```python
from build123d import *

# Parameters (mm, degrees)
F1_DEPTH = 40.2336
F0_R     = 10.16
F2_DEPTH = 15.7734
F3_R     = 3.302


# Not quite as in the source:
# - a feature names something its author has since deleted; it is built from what else it names


with BuildPart() as f1:
    # F0 (on Top) → F1 (new body)
    with BuildSketch(Plane.XY):
        with BuildLine():
            ThreePointArc((5.2118165727, -28.0956863773), (21.9710978739, -18.2702348977), (28.575, 0))
            ThreePointArc((28.575, 0), (21.9710978739, 18.2702348977), (5.2118165727, 28.0956863773))
            ThreePointArc((5.2118165727, 28.0956863773), (-28.575, 0), (5.2118165727, -28.0956863773))
        make_face()
        with BuildLine():
            ThreePointArc((13.4477648793, -4.826), (-14.2875, 0), (13.4477648793, 4.826))
            Line((13.4477648793, 4.826), (19.7977648793, 4.826))
            Line((19.7977648793, 4.826), (19.7977648793, -4.826))
            Line((19.7977648793, -4.826), (13.4477648793, -4.826))
        make_face(mode=Mode.SUBTRACT)
    extrude(amount=F1_DEPTH)

    # F0 (on Top) → F2 (join)
    with BuildSketch(Plane.XY):
        with BuildLine():
            ThreePointArc((5.2118165727, 28.0956863773), (21.9710978739, 18.2702348977), (28.575, 0))
            ThreePointArc((28.575, 0), (21.9710978739, -18.2702348977), (5.2118165727, -28.0956863773))
            Line((5.2118165727, -28.0956863773), (53.975, -19.05))
            ThreePointArc((53.975, -19.05), (34.925, 0), (53.975, 19.05))
            Line((53.975, 19.05), (5.2118165727, 28.0956863773))
        make_face()
        with BuildLine():
            ThreePointArc((73.025, 0), (67.4453841816, 13.4703841816), (53.975, 19.05))
            ThreePointArc((53.975, 19.05), (34.925, 0), (53.975, -19.05))
            ThreePointArc((53.975, -19.05), (67.4453841816, -13.4703841816), (73.025, 0))
        make_face()
        with Locations((53.975, 0)):
            Circle(F0_R, mode=Mode.SUBTRACT)
    extrude(amount=F2_DEPTH)

    # F3
    f3_edges = [f1.edges().sort_by_distance(p)[0] for p in [
        (-5.211817, 28.095686, 40.2336),
    ]]
    fillet(f3_edges, radius=F3_R)


solid = f1.part
```
Read the model definition and answer for the solid it produces. Units are mm, in the model's axes. A direction names the side the tool comes from. Coordinates: 2 decimals unless noted, no trailing zeros. Write each loop counter-clockwise with the first axis right and the second up, starting at its lowest first coordinate (ties: lowest second). Pieces come first, ordered by that corner, then holes. Notation, with made-up numbers: (12.5, 48) -> (31.5, 48) arc R19 ccw to (31.5, 60) -> close; hole circle Ø11 at (19.5, 85). An arc over 180 degrees is marked (long way). Write item = value, one per line.
(1) Which of the six approach directions +Z, -Z, +X, -X, +Y, -Y give full straight-line access (tool end or side, diameter ignored) to faces 4 (the face through (73.02, -0.42, 7.78)), 5 (the face through (19.798, 0, 20))?
From the geometry:
face_4 = +Z, -Z, +X
face_5 = +Z, -Z
(2) Straight lines are drawn through the part: L1, parallel to Y at x = 0, z = 25.5 (1 decimal); L2, parallel to X at y = 0, z = 28 (1 decimal); L3, parallel to X at y = 8.5, z = 6.5. For each, find the intervals that lie inside material, in ascending order. Write a range as from..to.
From the geometry:
L1 = -28.6..-14.3, 14.3..28.6
L2 = -28.6..-14.3, 19.8..28.6
L3 = -27.28..-11.48, 11.48..48.41, 59.54..71.02
(3) Section B-B on z = 3 is taken. Count the separate pieces of the cut face and the enclosed holes in it, plus the area to 3 significant figures.
From the geometry:
separate_pieces = 1
enclosed_holes = 2
area = 3,430 mm2
(4) Given pin 1 Ø3 at (y, z) = (0.5, 20) entering from -X (3 decimals); pin 2 Ø5 at (y, z) = (-3.5, 8.5) entering from +X; pin 3 Ø3 at (x, y) = (58, -18) entering from +Z; pin 4 Ø2 at (x, y) = (5, -10.5) entering from +Z, each flat-ended and moving along its own axis, determine where each tip first touches the part or whether it passes through.
From the geometry:
pin_1 = -28.575
pin_2 = 73
pin_3 = 15.77
pin_4 = through
(5) Section C-C on x = 66.5 is taken. Write down the section's boundary in (y, z), plus the area to 3 significant figures.
From the geometry:
outline = (-14.35, 0) -> (14.35, 0) -> (14.35, 15.77) -> (-14.35, 15.77) -> close
area = 453 mm2
(6) For a pull along X with two mould halves and no side action, classify faces 1 (the face through (29.93, 23.51, 7.78)), 2 (the face through (11, -11, 40.234)), 3 (the face through (17, 4.826, 20)) as +X half, -X half, draft (parallel to the pull), parting line (faces both ways), or undercut.
From the geometry:
face_1 = +X half
face_2 = draft
face_3 = undercut
